Check sheet for the drawn part. Datum: minimum x, y, z corner. Units: mm. Coordinates: 2 decimals unless noted, no trailing zeros. Write each loop counter-clockwise with the first axis right and the second up, starting at its lowest first coordinate (ties: lowest second). Pieces come first, ordered by that corner, then holes. Notation, with made-up numbers: M 56.25,-18.5 L 82.25,-18.5 A23 ccw 82.25,-4.5 Z; hole C 85.25,61.25 d10. An arc over 180 degrees is marked long. Answer as CSV lines item,"result". Start each with the question number.
Q1. Mould release check, pull along X, two halves, no side actions. Record for the marked faces 1, 2 and 3: pulls with the +X half, pulls with the -X half, needs draft (parallel to the pull), parting line crosses it, or undercut.
Q2. Sectioned sample at A-A, the plane y = 27.5. Record the cut outline in (x, z).
Q3. Sectioned sample at B-B, the plane x = 2.5. Record the cut outline in (y, z).
Q4. Sectioned sample at D-D, the plane z = 5.5. Record the cut outline in (x, y) (1 decimal).
Q5. Sectioned sample at C-C, the plane z = 1.5. Record the cut outline in (x, y).
Q6. Thickness scan on line 1 along Z through (x, y) = (3, 12.5) (1 decimal); line 2 along X through (y, z) = (20.25, 4.75) (1 decimal); line 3 along Z through (x, y) = (5.25, 20.25) (1 decimal). Record the ranges inside material, lowest first. Write a range as from..to.
Q7. Depth check by flat-ended pin: pin 1 Ø1 at (x, y) = (6, 9) entering from +Z (1 decimal); pin 2 Ø1.5 at (y, z) = (5, 4) entering from -X. Enter the tip coordinate at first touch or a pass-through.
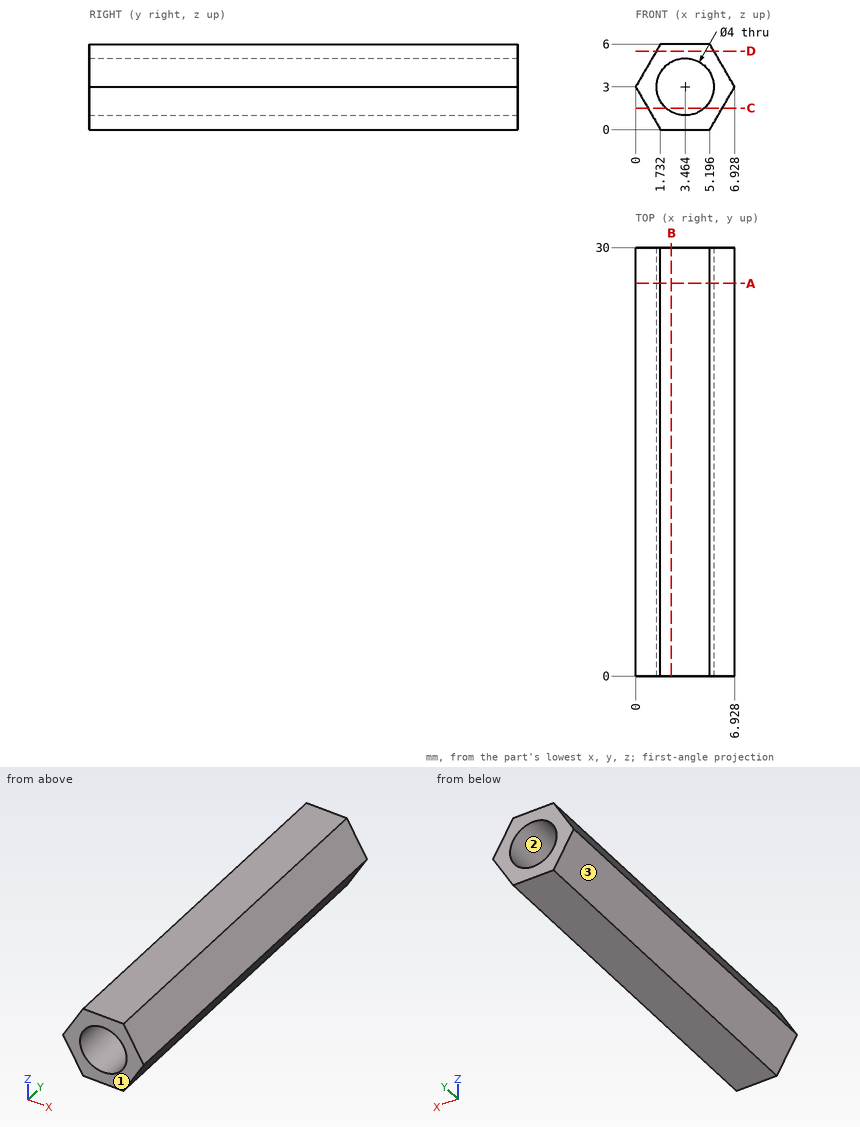
Output:
1,face 1,"needs draft"
1,face 2,"undercut"
1,face 3,"pulls with the -X half"
2,outline,"M 0,3 L 1.73,0 L 5.2,0 L 6.93,3 L 5.2,6 L 1.73,6 Z; hole C 3.46,3 d4"
3,outline,"M 0,0 L 30,0 L 30,1.25 L 0,1.25 Z; M 0,4.75 L 30,4.75 L 30,6 L 0,6 Z"
4,outline,"M 1.4,0 L 5.5,0 L 5.5,30 L 1.4,30 Z"
5,outline,"M 0.87,0 L 2.14,0 L 2.14,30 L 0.87,30 Z; M 4.79,0 L 6.06,0 L 6.06,30 L 4.79,30 Z"
6,line 1,"z = 0..1.1, 4.9..6"
6,line 2,"x = 1..2.5, 4.4..5.9"
6,line 3,"z = 0.1..2.1, 3.9..5.9"
7,pin 1,"stops at z = 5.5"
7,pin 2,"stops at x = 0.14"
